```python
from build123d import *

# Parameters (mm, degrees)
SKETCH2_R          = 4.5
CUT_EXTRUDE1_DEPTH = 0.1
CUT_EXTRUDE2_DEPTH = 0.1
SKETCH4_W          = 0.3
SKETCH4_H          = 2.5
FILLET1_R          = 0.5


with BuildPart() as part:
    # Sketch1 → Revolve1 (revolve)
    with BuildSketch(Plane.XY):
        with BuildLine():
            Line((5, 16), (0, 16))
            Line((0, 16), (0, 0))
            Line((0, 0), (4.827244523, 0))
            ThreePointArc((4.827244523, 0), (4.990681342, 0.249416346), (4.961933008, 0.546222076))
            ThreePointArc((4.961933008, 0.546222076), (4.887026856, 0.767683511), (4.861659937, 1.00008966))
            Line((4.861659937, 1.00008966), (4.861659937, 1.202915685))
            ThreePointArc((4.861659937, 1.202915685), (4.896669937, 1.431894531), (4.99850097, 1.639950899))
            ThreePointArc((4.99850097, 1.639950899), (4.999616482, 1.64223006), (5, 1.644738417))
            Line((5, 1.644738417), (5, 16))
        make_face()
    revolve(axis=Axis((0, 16, 0), (0, -1, 0)))

    # Sketch2 → Cut-Extrude1 (cut)
    with BuildSketch(Plane(origin=(0, 16, 0), x_dir=(-1, 0, 0), z_dir=(0, 1, 0))):
        with Locations(Location((0, 0, 0), (0, 0, 270))):
            Circle(SKETCH2_R)
    extrude(amount=-CUT_EXTRUDE1_DEPTH, mode=Mode.SUBTRACT)

    # Sketch3 → Cut-Extrude2 (cut)
    with BuildSketch(Plane(origin=(0, 15.9, 0), x_dir=(-1, 0, 0), z_dir=(0, 1, 0))):
        Polygon((2.906036622, -3.256093686), (3.090537324, -3.081521376), (0.142645036, 0.03402539), (1.320649975, 3.989641976), (1.07721557, 4.062138116), (-0.10078937, 0.10652153), (-4.155587963, -0.860677244), (-4.096654259, -1.107745693), (-0.041855666, -0.14054692), align=None)
    extrude(amount=-CUT_EXTRUDE2_DEPTH, mode=Mode.SUBTRACT)

    # Sketch4 → Revolve2 (revolve)
    with BuildSketch(Plane(origin=(0, 0, 0), x_dir=(-1, 0, 0), z_dir=(0, 0, -1)), mode=Mode.PRIVATE) as revolve2_sk:
        with Locations((-2.65, -1.25)):
            Rectangle(SKETCH4_W, SKETCH4_H)
    revolve2 = revolve(revolve2_sk.sketch.rotate(Axis((2.5, -2.5, 0), (0, 1, 0)), 270), axis=Axis((2.5, -2.5, 0), (0, 1, 0)))

    # Fillet1
    fillet1_edges = [part.edges().sort_by_distance(p)[0] for p in [
        (-5, 16, 0),
        (-4.827244523, 0, 0),
    ]]
    fillet(fillet1_edges, radius=FILLET1_R - 0.0001)  # a hair under: the kernel refuses the full size

    # Simetría3: Revolve2 across plane
    add(revolve2.mirror(Plane(origin=(0, 0, 0), x_dir=(0, 0, 1), z_dir=(1, 0, 0))))


solid = part.part
```
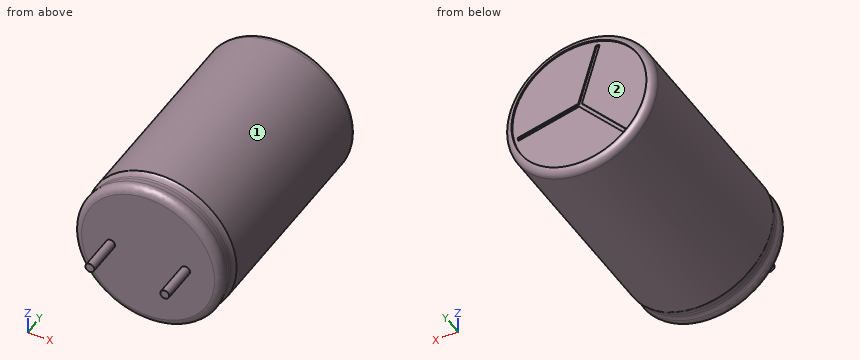
Geometry check sheet. Reference: the model listing, model coordinates, mm. Face numbers are marked on the shaded views. Give positions to 0.01 mm unless a question says otherwise; leave off trailing zeros. Write each loop counter-clockwise with the first axis right and the second up, starting at its lowest first coordinate (ties: lowest second). Pieces come first, ordered by that corner, then holes. Notation, with made-up numbers: (61.5, 0) -> (116.5, 0) arc R22 cw to (116.5, 17) -> close; hole circle Ø3 at (77.25, -5.75). An arc over 180 degrees is marked (long way). One line per question, with ' | ' between items.
Item 1: Sectioned sample at A-A, the plane y = 15.25. Record the boundary of the cut face in (x, z), plus the area to 3 significant figures.
Determined:
outline: circle Ø10 at (0, 0) | area: 78.5 mm^2
Item 2: Draft check along X on the marked faces 1 and 2. Enter one of: released by +X, released by -X, zero draft, split by the parting line, or undercut.
Determined:
face 1: split by the parting line | face 2: undercut
Item 3: Depth check by flat-ended pin: pin 1 (1 mm diameter, centred on x = -2, z = -4, fed in from -Y); pin 2 (4 mm diameter, centred on y = -0.5, z = 2.5, fed in from -X); pin 3 (2 mm diameter, centred on x = 1, z = -1.5, fed in from +Y). Enter the tip coordinate at first touch or a pass-through.
Determined:
pin 1: y = 0 | pin 2: x = -4.88 | pin 3: y = 15.9
Item 4: Scan lines: line 1 along Y through (x, z) = (-3, -0.25); line 2 along Y through (x, z) = (-2.25, 0); line 3 along X through (y, z) = (3, -0.25). Record each from-to range of solid material in increasing order.
Determined:
line 1: 0 to 15.9 | line 2: -2.5 to 15.9 | line 3: -4.99 to 4.99
